from build123d import *

# Parameters (mm, degrees)
EXTRUDE_1_DEPTH     = 1
FILLET_1_R          = 10
FILLET_2_R          = 8
SKETCH_2_R          = 5.5
CUT_EXTRUDE_1_DEPTH = 10


with BuildPart() as part:
    # Эскиз1 → Бобышка-Вытянуть1 (new, symmetric)
    with BuildSketch(Plane.XY):
        Polygon((-210, 155), (-210, 190), (210, 190), (210, 155), (218, 155), (218, -155), (210, -155), (210, -190), (-210, -190), (-210, -155), (-218, -155), (-218, 155), align=None)
    extrude(amount=EXTRUDE_1_DEPTH, both=True)

    # Скругление1
    fillet_1_edges = [part.edges().sort_by_distance(p)[0] for p in [
        (210, -190, 0),
        (-210, -190, 0),
        (-210, 190, 0),
        (210, 190, 0),
    ]]
    fillet(fillet_1_edges, radius=FILLET_1_R)

    # Скругление2
    fillet_2_edges = [part.edges().sort_by_distance(p)[0] for p in [
        (-218, -155, 0),
        (-218, 155, 0),
        (218, 155, 0),
        (218, -155, 0),
    ]]
    fillet(fillet_2_edges, radius=FILLET_2_R - 0.0001)  # a hair under: the kernel refuses the full size

    # Эскиз2 → Вырез-Вытянуть1 (cut)
    with BuildSketch(Plane.XY.offset(1)):
        with Locations((0, -172)):
            Circle(SKETCH_2_R)
        with Locations((152, -172)):
            Circle(SKETCH_2_R)
        with Locations((-152, -172)):
            Circle(SKETCH_2_R)
        with Locations((-152, 172)):
            Circle(SKETCH_2_R)
        with Locations((152, 172)):
            Circle(SKETCH_2_R)
        with Locations((0, 172)):
            Circle(SKETCH_2_R)
    extrude(amount=-CUT_EXTRUDE_1_DEPTH, mode=Mode.SUBTRACT)


solid = part.part
Model file for the job. Use its own axes, mm. Coordinates: 2 decimals unless noted, no trailing zeros. Write each loop counter-clockwise with the first axis right and the second up, starting at its lowest first coordinate (ties: lowest second). Pieces come first, ordered by that corner, then holes. Notation, with made-up numbers: (61.25, -30) -> (95.25, -30) arc R31 ccw to (95.25, 0) -> close; hole circle Ø11 at (45.5, 61). An arc over 180 degrees is marked (long way). One line per item, written item: value. Start each with the question number.
1) Slice it at B-B on x = 152. Write the cut outline in (y, z), then the cut area to 3 significant figures.
2) Pull direction Y, two halves, no side cores. Call faces 1 (the face through (-207.15, -186.99, -0.01)), 2 (the face through (207.15, 186.99, -0.01)), 3 (the face through (146.505, -171.758, 0.014)), 4 (the face through (3, 3, 1)): +Y half, -Y half, draft (parallel to the pull), parting line (faces both ways), or undercut.
3) Slice it at A-A on y = 172. Write the cut outline in (x, z), then the cut area to 3 significant figures.
4) Probe probe 1 along Y at (x, z) = (-152, -0.2); probe 2 along Y at (x, z) = (-156, 0.95). List the from-to ranges inside material, lowest first.
5) Flat gauge pins, fed straight in: pin 1 Ø1 at (y, z) = (-168, 0.5) entering from +X; pin 2 Ø12.5 at (x, y) = (152, 172) entering from -Z; pin 3 Ø0.6 at (y, z) = (-164, -0.5) entering from -X. Where does each tip first touch, or does it go through?
Answers follow:
1. outline: (-190, -1) -> (-177.5, -1) -> (-177.5, 1) -> (-190, 1) -> close; (-166.5, -1) -> (166.5, -1) -> (166.5, 1) -> (-166.5, 1) -> close; (177.5, -1) -> (190, -1) -> (190, 1) -> (177.5, 1) -> close
1. area: 716 mm2
2. face 1: -Y half
2. face 2: +Y half
2. face 3: undercut
2. face 4: draft
3. outline: (-210, -1) -> (-157.5, -1) -> (-157.5, 1) -> (-210, 1) -> close; (-146.5, -1) -> (-5.5, -1) -> (-5.5, 1) -> (-146.5, 1) -> close; (5.5, -1) -> (146.5, -1) -> (146.5, 1) -> (5.5, 1) -> close; (157.5, -1) -> (210, -1) -> (210, 1) -> (157.5, 1) -> close
3. area: 774 mm2
4. probe 1: -190 to -177.5, -166.5 to 166.5, 177.5 to 190
4. probe 2: -190 to -175.77, -168.23 to 168.23, 175.77 to 190
5. pin 1: x = 210
5. pin 2: z = -1
5. pin 3: x = -210
